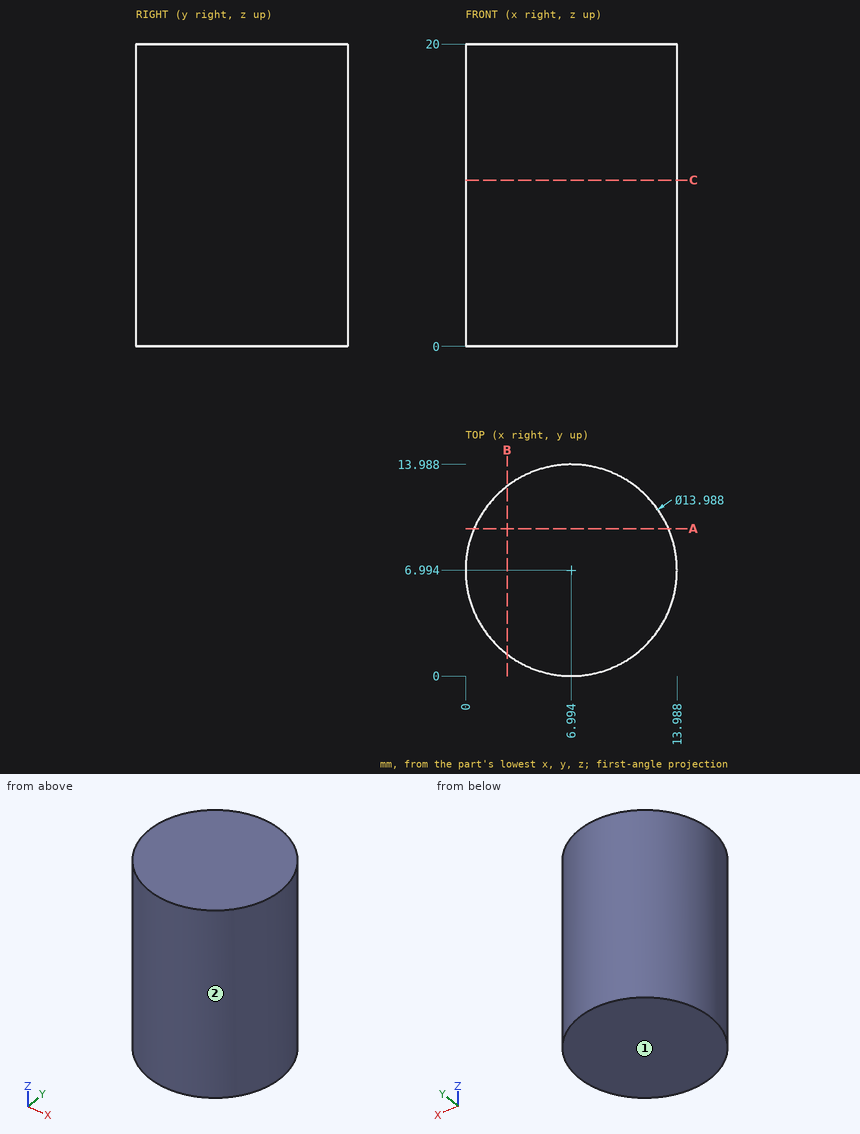
Check sheet for the drawn part. Datum: minimum x, y, z corner. Units: mm. Round coordinates to 2 decimals unless told otherwise and drop trailing zeros. Loops run counter-clockwise (first coordinate to the right, second up) from the corner with the lowest first, then second, coordinate; pieces in that order, holes last. Notation, with made-up numbers: (44, 24) - (67, 24) arc R17 cw to (67, 34) - close; hole circle Ø4 at (51, 66.5). An arc over 180 degrees is marked (long way). Answer as a JSON object with one key per item and string values. Group by question number.
Q1. Sectioned sample at B-B, the plane x = 2.75. Enter the section's corners in (y, z) (1 decimal).
Q2. Sectioned sample at C-C, the plane z = 11. Enter the section's corners in (x, y).
Q3. Mould release check, pull along Y, two halves, no side actions. Record for the marked faces 1 and 2: released by +Y, released by -Y, zero draft, split by the parting line, or undercut.
Q4. Sectioned sample at A-A, the plane y = 9.75. Enter the section's corners in (x, z).
Q5. Scan lines: line 1 along Y through (x, z) = (8, 6.75) (1 decimal); line 2 along Y through (x, z) = (7.5, 14); line 3 along X through (y, z) = (2, 11). Record each from-to range of solid material in increasing order. Write a range as [from, to].
Q6. Gauge pin test, flat ends, axial feed: P1, Ø5, axis at x = 3.5, z = 16.5, coming from the +Y side; P2, Ø1.5, axis at y = 2.5, z = 14, coming from the -X side. Record the tip position at first contact, or that the pin passes through.
Solution:
{
 "1": {"outline": "(1.4, 0) - (12.6, 0) - (12.6, 20) - (1.4, 20) - close"},
 "2": {"outline": "circle Ø13.99 at (6.99, 6.99)"},
 "3": {"face 1": "zero draft", "face 2": "split by the parting line"},
 "4": {"outline": "(0.57, 0) - (13.42, 0) - (13.42, 20) - (0.57, 20) - close"},
 "5": {"line 1": "y = [0.1, 13.9]", "line 2": "y = [0.02, 13.97]", "line 3": "x = [2.1, 11.89]"},
 "6": {"P1": "stops at y = 13.92", "P2": "stops at x = 1.09"}
}
